from build123d import *

# Parameters (mm, degrees)
EXTRUDE_1_DEPTH     = 150
SKETCH_2_W          = 160
SKETCH_2_H          = 60
EXTRUDE_2_DEPTH     = 4
SKETCH_3_W          = 160
SKETCH_3_H          = 60
EXTRUDE_3_DEPTH     = 4
EXTRUDE_5_DEPTH     = 150
SKETCH_8_W          = 30
SKETCH_8_H          = 4
EXTRUDE_6_DEPTH     = 150
CUT_EXTRUDE_1_REACH = 272.328
SKETCH_10_R         = 10
CUT_EXTRUDE_2_DEPTH = 10
SKETCH_11_R         = 5
CUT_EXTRUDE_3_DEPTH = 10


with BuildPart() as part:
    # 草图1 → 凸台-拉伸1 (new body)
    with BuildSketch(Plane(origin=(0, 0, 0), x_dir=(0, 0, -1), z_dir=(1, 0, 0))):
        Polygon((30, 31), (30, 0), (0, 0), (0, -4), (30, -4), (30, -29), (190, -29), (190, 27.892594103), (186, 27.892594103), (186, -25), (98, -25), (98, 31), (94, 31), (94, -25), (34, -25), (34, 31), align=None)
    extrude(amount=EXTRUDE_1_DEPTH)

    # 草图2 → 凸台-拉伸2 (add)
    with BuildSketch(Plane(origin=(150, 0, 0), x_dir=(0, 0, -1), z_dir=(1, 0, 0))):
        with Locations((110, 1)):
            Rectangle(SKETCH_2_W, SKETCH_2_H)
    extrude(amount=EXTRUDE_2_DEPTH)

    # 草图3 → 凸台-拉伸3 (add)
    with BuildSketch(Plane.ZY):
        with Locations((-110, 1)):
            Rectangle(SKETCH_3_W, SKETCH_3_H)
    extrude(amount=EXTRUDE_3_DEPTH)

    # 草图5 → 凸台-拉伸5 (add)
    with BuildSketch(Plane(origin=(150, 0, -30), x_dir=(0, 0, 1), z_dir=(-1, 0, 0))):
        with BuildLine():
            add(Edge.make_bspline(
                [(0, 18.235042401), (2.837739177, 7.092842101), (9.238577647, 0)],
                knots=[0, 0, 0, 1, 1, 1], degree=2))
            Line((9.238577647, 0), (9.33878145, -0.092906558))
            Line((9.33878145, -0.092906558), (0, 0))
            Line((0, 0), (0, 18.235042401))
        make_face()
        with BuildLine():
            Line((0, -4), (0, -16.851035139))
            add(Edge.make_bspline(
                [(0, -16.851035139), (3.667477497, -10.331662623), (9.475645739, -4)],
                knots=[0, 0, 0, 1, 1, 1], degree=2))
            Line((9.475645739, -4), (0, -4))
        make_face()
    extrude_5 = extrude(amount=EXTRUDE_5_DEPTH)

    # 镜向2: 凸台-拉伸5 across plane
    add(extrude_5.mirror(Plane.XY.offset(-110)))

    # 草图8 → 凸台-拉伸6 (add)
    with BuildSketch(Plane(origin=(150, 0, 0), x_dir=(0, 0, -1), z_dir=(1, 0, 0))):
        with Locations((205, -2)):
            Rectangle(SKETCH_8_W, SKETCH_8_H)
    extrude(amount=-EXTRUDE_6_DEPTH)

    # 草图9 → 切除-拉伸1 (cut, up to next)
    with BuildSketch(Plane(origin=(150, 0, 0), x_dir=(0, 0, -1), z_dir=(1, 0, 0)), mode=Mode.PRIVATE) as cut_extrude_1_sk1:
        Polygon((199.475645739, -4), (190, -4), (190, -16.851035139), align=None)
    cut_extrude_1_tool1 = extrude(cut_extrude_1_sk1.sketch, amount=-CUT_EXTRUDE_1_REACH, mode=Mode.PRIVATE) & part.part
    add(cut_extrude_1_tool1.solids().sort_by_distance((150, -8.283678, -193.158549))[0], mode=Mode.SUBTRACT)

    # 草图10 → 切除-拉伸2 (cut)
    with BuildSketch(Plane(origin=(0, 0, -98), x_dir=(-1, 0, 0), z_dir=(0, 0, -1))):
        with Locations(Location((-137.288939056, 2.62555121, 0), (0, 0, 90))):
            Circle(SKETCH_10_R)
    extrude(amount=-CUT_EXTRUDE_2_DEPTH, mode=Mode.SUBTRACT)

    # 草图11 → 切除-拉伸3 (cut)
    with BuildSketch(Plane.XY.offset(-30)):
        with Locations((134.999120895, 24.559728505)):
            Circle(SKETCH_11_R)
    extrude(amount=-CUT_EXTRUDE_3_DEPTH, mode=Mode.SUBTRACT)


solid = part.part
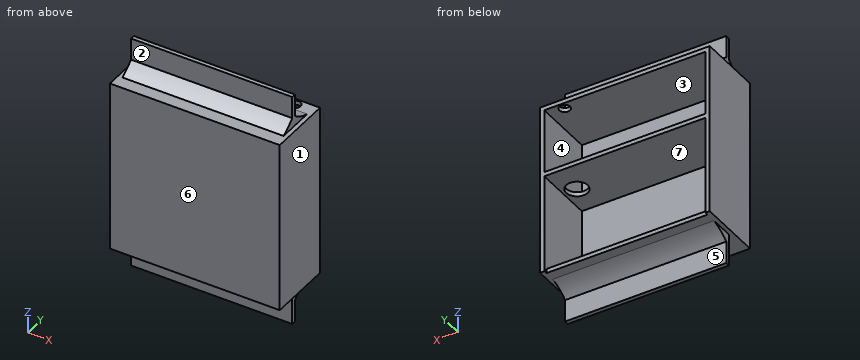
Geometry: final body of the model. Coordinates: model frame, mm. Face numbers are marked on the shaded views. A direction names the side the tool comes from. Round coordinates to 2 decimals unless told otherwise and drop trailing zeros. Order: outer loops, then holes, each group sorted by start corner. A loop starts at its lowest first (then second) coordinate and runs counter-clockwise, first axis right, second up.
Q1. Section B-B, the plane y = -20. Output: boundary loops of the cut face in (x, z).
Result sheet:
outline: (-4, -190) - (154, -190) - (154, -30) - (-4, -30) - close; hole (0, -186) - (150, -186) - (150, -98) - (0, -98) - close; hole (0, -94) - (150, -94) - (150, -34) - (0, -34) - close
Q2. Mould query, pull axis X, two halves, no side actions, for the marked faces 1, 2, 3 and 4. Classes: released by +X, released by -X, zero draft, split by the parting line, or undercut.
Result sheet:
face 1: released by +X
face 2: zero draft
face 3: undercut
face 4: undercut
Q3. Section C-C, the plane y = 22. Output: boundary loops of the cut face in (x, z), and give its area (3 significant figures).
Result sheet:
outline: (-4, -190) - (154, -190) - (154, -30) - (139.29, -30) - (139.29, -34) - (150, -34) - (150, -94) - (0, -94) - (0, -34) - (130.7, -34) - (130.7, -30) - (-4, -30) - close; hole (0, -186) - (150, -186) - (150, -98) - (0, -98) - close
area: 3,050 mm2
Q4. Access query for the marked faces 5, 6 and 7. Directions: +Z, -Z, +X, -X, +Y, -Y. A direction counts if a zero-diameter tool reaches every point of the face in a straight line with its end or side. Return the directions, or none.
Result sheet:
face 5: -Z, +X, -X, +Y
face 6: +Z, -Z, +X, -X, -Y
face 7: +Y
Q5. Pin query (flat end, axial travel): pin 1 (6 mm diameter, centred on x = 89, z = -15, fed in from -Y); pin 2 (10.5 mm diameter, centred on x = 72.5, z = -207, fed in from +Y); pin 3 (6.5 mm diameter, centred on y = 4, z = -205.5, fed in from -X); pin 4 (16 mm diameter, centred on x = 53, y = 14.5, fed in from +Z). Return the tip coordinate at first contact, or that it passes through.
Result sheet:
pin 1: stops at y = -4
pin 2: stops at y = 0
pin 3: passes through
pin 4: stops at z = -25.41
Q6. Material intervals for probe 1 along Z at (x, y) = (42, -23); probe 2 along Z at (x, y) = (118, 7); probe 3 along X at (y, z) = (-8.5, -148), sorted ascending.
Result sheet:
probe 1: z = -190 to -186, -98 to -94, -34 to -30
probe 2: z = -194.31 to -186, -98 to -94, -34 to -25.69
probe 3: x = -4 to 0, 150 to 154
Q7. Section D-D, the plane z = -204. Output: boundary loops of the cut face in (x, y).
Result sheet:
outline: (0, -4) - (150, -4) - (150, 0) - (0, 0) - close
Q8. Section A-A, the plane z = -79. Output: boundary loops of the cut face in (x, y).
Result sheet:
outline: (-4, -29) - (154, -29) - (154, 31) - (150, 31) - (150, -25) - (0, -25) - (0, 31) - (-4, 31) - close
